from build123d import *

# Parameters (mm, degrees)
EXTRUDE_1_DEPTH = 3


with BuildPart() as part:
    # Эскиз1 → Бобышка-Вытянуть1 (new body)
    with BuildSketch(Plane(origin=(0, 0, 0), x_dir=(1, 0, 0), z_dir=(0, 1, 0))):
        Polygon((4.6, 70), (4.6, 73), (10, 73), (10, 70), (14.6, 70), (14.6, 73), (20, 73), (20, 70), (24.6, 70), (24.6, 73), (30, 73), (30, 70), (34.6, 70), (34.6, 73), (40, 73), (40, 70), (44.6, 70), (44.6, 73), (50, 73), (50, 70), (54.6, 70), (54.6, 73), (60, 73), (60, 70), (64.6, 70), (64.6, 73), (70, 73), (70, 70), (74.6, 70), (74.6, 73), (80, 73), (80, 70), (84.6, 70), (84.6, 73), (90, 73), (90, 70), (94.6, 70), (94.6, 73), (100, 73), (100, 70), (104.6, 70), (104.6, 73), (110, 73), (110, 70), (114.6, 70), (114.6, 73), (120, 73), (120, 70), (124.6, 70), (124.6, 73), (130, 73), (130, 70), (134.6, 70), (134.6, 73), (140, 73), (140, 70), (144.6, 70), (144.6, 73), (150, 73), (150, 70), (154.6, 70), (154.6, 73), (160, 73), (160, 70), (164.6, 70), (164.6, 65.4), (167.6, 65.4), (167.6, 60), (164.6, 60), (164.6, 55.4), (167.6, 55.4), (167.6, 50), (164.6, 50), (164.6, 45.4), (167.6, 45.4), (167.6, 40), (164.6, 40), (164.6, 35.4), (167.6, 35.4), (167.6, 30), (164.6, 30), (164.6, 25.4), (167.6, 25.4), (167.6, 20), (164.6, 20), (164.6, 15.4), (167.6, 15.4), (167.6, 10), (164.6, 10), (164.6, 5.4), (167.6, 5.4), (167.6, -3), (164.6, -3), (164.6, 0), (160, 0), (160, -3), (154.6, -3), (154.6, 0), (150, 0), (150, -3), (144.6, -3), (144.6, 0), (140, 0), (140, -3), (134.6, -3), (134.6, 0), (130, 0), (130, -3), (124.6, -3), (124.6, 0), (120, 0), (120, -3), (114.6, -3), (114.6, 0), (110, 0), (110, -3), (104.6, -3), (104.6, 0), (100, 0), (100, -3), (94.6, -3), (94.6, 0), (90, 0), (90, -3), (84.6, -3), (84.6, 0), (80, 0), (80, -3), (74.6, -3), (74.6, 0), (70, 0), (70, -3), (64.6, -3), (64.6, 0), (60, 0), (60, -3), (54.6, -3), (54.6, 0), (50, 0), (50, -3), (44.6, -3), (44.6, 0), (40, 0), (40, -3), (34.6, -3), (34.6, 0), (30, 0), (30, -3), (24.6, -3), (24.6, 0), (20, 0), (20, -3), (14.6, -3), (14.6, 0), (10, 0), (10, -3), (4.6, -3), (4.6, 0), (0, 0), (0, -3), (-3, -3), (-3, 5.4), (0, 5.4), (0, 10), (-3, 10), (-3, 15.4), (0, 15.4), (0, 20), (-3, 20), (-3, 25.4), (0, 25.4), (0, 30), (-3, 30), (-3, 35.4), (0, 35.4), (0, 40), (-3, 40), (-3, 45.4), (0, 45.4), (0, 50), (-3, 50), (-3, 55.4), (0, 55.4), (0, 60), (-3, 60), (-3, 65.4), (0, 65.4), (0, 70), align=None)
    extrude(amount=EXTRUDE_1_DEPTH)


solid = part.part
Verification items for the finished model (mm, model axes). A direction names the side the tool comes from. Coordinates: 2 decimals unless noted, no trailing zeros. Order: outer loops, then holes, each group sorted by start corner. A loop starts at its lowest first (then second) coordinate and runs counter-clockwise, first axis right, second up.
1. Sectioned sample at A-A, the plane x = 21.5. Record the cut outline in (y, z).
Results found:
outline: (0, -70) - (3, -70) - (3, 0) - (0, 0) - close
2. Go/stop test with flat-tipped pins: pin 1 Ø0.9 at (y, z) = (1, -71) entering from -X; pin 2 Ø0.9 at (x, y) = (142.5, 1.5) entering from -Z; pin 3 Ø1.5 at (y, z) = (2, -7.5) entering from -X. Record where each tip stops, or that it passes through.
Results found:
pin 1: stops at x = 4.6
pin 2: stops at z = -70
pin 3: stops at x = 0
3. Release check for a two-part mould opening along X. For faces 1 (the face through (94.6, 1, 2)), 2 (the face through (160, 1, -72)), 3 (the face through (-3, 1, -33)), 4 (the face through (166, 1, 3)) record: +X half, -X half, draft (parallel to the pull), parting line (faces both ways), or undercut.
Results found:
face 1: undercut
face 2: +X half
face 3: -X half
face 4: draft
4. Set-up check for faces 5 (the face through (20, 1, -72)), 6 (the face through (2, 1, -70)), 7 (the face through (0, 1, -18)), 8 (the face through (164.6, 1, -68)): record each of +Z, -Z, +X, -X, +Y, -Y from which the full face is reachable in a straight line by a thin tool's end or side.
Results found:
face 5: -Z, +Y, -Y
face 6: -Z, -X, +Y, -Y
face 7: -X, +Y, -Y
face 8: -Z, +X, +Y, -Y
5. Sectioned sample at B-B, the plane z = -8.5. Record the cut outline in (x, y).
Results found:
outline: (0, 0) - (164.6, 0) - (164.6, 3) - (0, 3) - close
6. Scan lines: line 1 (X direction, y = 0.2, z = -68); line 2 (Z direction, x = 101.5, y = 2.65). Record each from-to range of solid material in increasing order.
Results found:
line 1: x = 0 to 164.6
line 2: z = -70 to 0
